```python
from build123d import *

# Parameters (mm, degrees)
BOSS_EXTRUDE1_DEPTH     = 75
FILLET1_R               = 5
CUT_EXTRUDE1_DEPTH      = 3.701539391
CUT_EXTRUDE1_DEPTH_BACK = 13.5
CUT_EXTRUDE2_DEPTH      = 1
CUT_EXTRUDE2_DEPTH_BACK = 176
SKETCH4_W               = 4.43767441
SKETCH4_H               = 75
BOSS_EXTRUDE2_DEPTH     = 15


with BuildPart() as part:
    # Sketch1 → Boss-Extrude1 (new body)
    with BuildSketch(Plane(origin=(0, 0, 0), x_dir=(1, 0, 0), z_dir=(0, 1, 0))):
        with BuildLine():
            Line((-87.5, 2.5), (-87.5, 12.5))
            Line((-87.5, 12.5), (87.5, 12.5))
            Line((87.5, 12.5), (87.5, 2.5))
            ThreePointArc((87.5, 2.5), (0, -2.701539391), (-87.5, 2.5))
        make_face()
    extrude(amount=BOSS_EXTRUDE1_DEPTH)

    # Fillet1
    fillet1_edges = [part.edges().sort_by_distance(p)[0] for p in [
        (-87.5, 37.5, -2.5),
        (87.5, 37.5, -2.5),
    ]]
    fillet(fillet1_edges, radius=FILLET1_R)

    # Sketch2 → Cut-Extrude1 (cut, two sides)
    with BuildSketch(Plane.XY) as cut_extrude1_sk:
        with BuildLine():
            Line((-83.06232559, 63), (-83.06232559, 0))
            Line((-83.06232559, 0), (83.06232559, 0))
            Line((83.06232559, 0), (83.06232559, 63))
            ThreePointArc((83.06232559, 63), (0, 60), (-83.06232559, 63))
        make_face()
    extrude(amount=CUT_EXTRUDE1_DEPTH, mode=Mode.SUBTRACT)
    extrude(cut_extrude1_sk.sketch, amount=-CUT_EXTRUDE1_DEPTH_BACK, mode=Mode.SUBTRACT)

    # Sketch3 → Cut-Extrude2 (cut, two sides)
    with BuildSketch(Plane.ZY.offset(87.5)) as cut_extrude2_sk:
        with BuildLine():
            Line((-1.984131445, 63), (-1.984131445, 8))
            ThreePointArc((-1.984131445, 8), (-3.484131445, 35.5), (-1.984131445, 63))
        make_face()
    extrude(amount=CUT_EXTRUDE2_DEPTH, mode=Mode.SUBTRACT)
    extrude(cut_extrude2_sk.sketch, amount=-CUT_EXTRUDE2_DEPTH_BACK, mode=Mode.SUBTRACT)

    # Sketch4 → Boss-Extrude2 (add)
    with BuildSketch(Plane(origin=(0, 0, -12.5), x_dir=(-1, 0, 0), z_dir=(0, 0, -1))):
        with Locations((-85.281162795, 37.5)):
            Rectangle(SKETCH4_W, SKETCH4_H)
        with Locations((85.281162795, 37.5)):
            Rectangle(SKETCH4_W, SKETCH4_H)
    extrude(amount=BOSS_EXTRUDE2_DEPTH)


solid = part.part
```
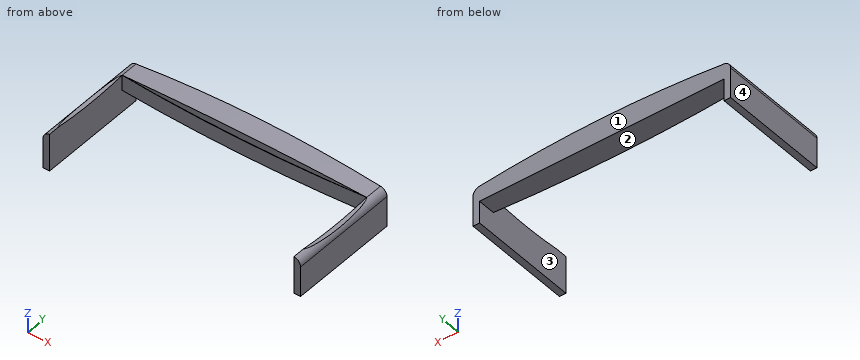
Can you work these out from the model? Positions are in its coordinate system, mm. Face numbers are marked on the shaded views. Coordinates: 2 decimals unless noted, no trailing zeros. Loops run counter-clockwise (first coordinate to the right, second up) from the corner with the lowest first, then second, coordinate; pieces in that order, holes last. Notation, with made-up numbers: (85.5, -2.5) - (115.5, -2.5) arc R23 ccw to (115.5, 21.5) - close; hole circle Ø8 at (34.5, -37). An arc over 180 degrees is marked (long way). Use a Markdown table: item, result.
Item 1: I want a section at A-A on y = 70. Please give me the cut outline in (x, z), and give its area (3 significant figures).
Numbers:
| item | result |
|---|---|
| outline | (-87.5, -27.5) - (-83.06, -27.5) - (-83.06, -12.5) - (83.06, -12.5) - (83.06, -27.5) - (87.5, -27.5) - (87.5, -6.95) arc R5 ccw to (83.06, -1.98) arc R738.56 ccw to (-83.06, -1.98) arc R5 ccw to (-87.5, -6.95) - close |
| area | 2,480 mm2 |
Item 2: We'd pull the mould along X, two halves only. Please class the marked faces 1, 2, 3 and 4: released by +X, released by -X, zero draft, split by the parting line, or undercut.
Numbers:
| item | result |
|---|---|
| face 1 | zero draft |
| face 2 | undercut |
| face 3 | undercut |
| face 4 | released by -X |
Item 3: I want a section at C-C on y = 21.5. Please give me the cut outline in (x, z).
Numbers:
| item | result |
|---|---|
| outline | (-87.5, -27.5) - (-83.06, -27.5) - (-83.06, -3.1) - (-85.68, -3.1) arc R5 ccw to (-87.5, -6.95) - close; (83.06, -27.5) - (87.5, -27.5) - (87.5, -6.95) arc R5 ccw to (85.68, -3.1) - (83.06, -3.1) - close |
Item 4: I want a section at B-B on z = -22. Please give me the cut outline in (x, y), and give its area (3 significant figures).
Numbers:
| item | result |
|---|---|
| outline | (-87.5, 0) - (-83.06, 0) - (-83.06, 75) - (-87.5, 75) - close; (83.06, 0) - (87.5, 0) - (87.5, 75) - (83.06, 75) - close |
| area | 666 mm2 |
Item 5: If I drill on probe 1 along X at (y, z) = (27, -20.5); probe 2 along Y at (x, z) = (-6.5, -9.5); probe 3 along X at (y, z) = (5.5, -6), over which ranges is the centre line in solid material (lowest first)? Write a range as from..to.
Numbers:
| item | result |
|---|---|
| probe 1 | x = -87.5..-83.06, 83.06..87.5 |
| probe 2 | y = 60.02..75 |
| probe 3 | x = -87.41..-83.06, 83.06..87.41 |
Item 6: I want a section at D-D on x = -76. Please give me the cut outline in (y, z), and give its area (3 significant figures).
Numbers:
| item | result |
|---|---|
| outline | (62.51, -12.5) - (75, -12.5) - (75, -1.22) - (62.51, -1.22) - (62.51, -1.98) - (63, -1.98) arc R252.83 cw to (62.51, -2.04) - close |
| area | 141 mm2 |
Item 7: Will these pins go through, and if not, where does the flat tip stop? pin 1 (2.5 mm diameter, centred on x = -30.5, y = 62, fed in from -Z); pin 2 (1 mm diameter, centred on y = 48.5, z = -6, fed in from +X); pin 3 (1 mm diameter, centred on y = 25.5, z = -5, fed in from +X).
Numbers:
| item | result |
|---|---|
| pin 1 | stops at z = -12.5 |
| pin 2 | stops at x = 87.48 |
| pin 3 | stops at x = 87.28 |
